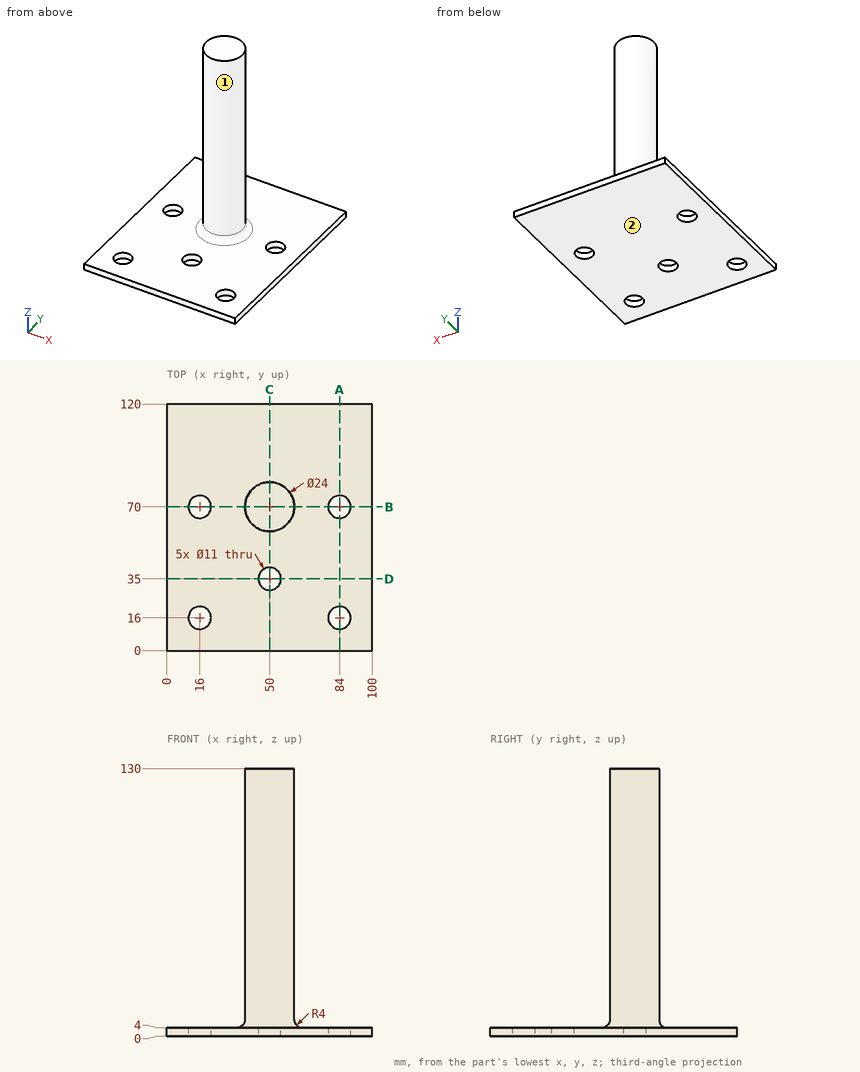
Geometry check sheet. Reference: drawing and pictorial views, mm from the part's lowest x, y, z. A direction names the side the tool comes from. Give positions to 0.01 mm unless a question says otherwise; leave off trailing zeros. Write each loop counter-clockwise with the first axis right and the second up, starting at its lowest first coordinate (ties: lowest second). Pieces come first, ordered by that corner, then holes.
Item 1: Cross-section at C-C (x = 50). Enter the section's corners in (y, z), and give its area (3 significant figures).
Item 2: Cross-section at B-B (y = 70). Enter the section's corners in (x, z), and give its area (3 significant figures).
Item 3: Access from +Z, -Z, +X, -X, +Y, -Y to the whole of each face (thin tool, end or side, straight path). Record for the marked faces 1 and 2.
Item 4: Scan lines: L1, parallel to Y at x = 84, z = 1.4; L2, parallel to Y at x = 50, z = 2; L3, parallel to Z at x = 32.5, y = 35.5. Record each from-to range of solid material in increasing order.
Item 5: Cross-section at D-D (y = 35). Enter the section's corners in (x, z).
Item 6: Cross-section at A-A (x = 84). Enter the section's corners in (y, z), and give its area (3 significant figures).
Item 7: Gauge pin test, flat ends, axial feed: pin 1 (14.5 mm diameter, centred on x = 50, y = 35, fed in from +Z); pin 2 (1 mm diameter, centred on y = 81.5, z = 31, fed in from -X); pin 3 (5 mm diameter, centred on x = 32.5, y = 13.5, fed in from -Z); pin 4 (5 mm diameter, centred on x = 40.5, y = 56, fed in from +Z). Record the tip position at first contact, or that the pin passes through.
Report:
1. outline: (0, 0) - (29.5, 0) - (29.5, 4) - (0, 4) - close; (40.5, 0) - (120, 0) - (120, 4) - (86, 4) arc R4 cw to (82, 8) - (82, 130) - (58, 130) - (58, 8) arc R4 cw to (54, 4) - (40.5, 4) - close
1. area: 3,470 mm2
2. outline: (0, 0) - (10.5, 0) - (10.5, 4) - (0, 4) - close; (21.5, 0) - (78.5, 0) - (78.5, 4) - (66, 4) arc R4 cw to (62, 8) - (62, 130) - (38, 130) - (38, 8) arc R4 cw to (34, 4) - (21.5, 4) - close; (89.5, 0) - (100, 0) - (100, 4) - (89.5, 4) - close
2. area: 3,340 mm2
3. face 1: +Z
3. face 2: -Z, +X, -X, +Y, -Y
4. L1: y = 0 to 10.5, 21.5 to 64.5, 75.5 to 120
4. L2: y = 0 to 29.5, 40.5 to 120
4. L3: z = 0 to 4
5. outline: (0, 0) - (44.5, 0) - (44.5, 4) - (0, 4) - close; (55.5, 0) - (100, 0) - (100, 4) - (55.5, 4) - close
6. outline: (0, 0) - (10.5, 0) - (10.5, 4) - (0, 4) - close; (21.5, 0) - (64.5, 0) - (64.5, 4) - (21.5, 4) - close; (75.5, 0) - (120, 0) - (120, 4) - (75.5, 4) - close
6. area: 392 mm2
7. pin 1: stops at z = 4
7. pin 2: stops at x = 45.2
7. pin 3: stops at z = 0
7. pin 4: stops at z = 4.33
